Can you work these out from the model? Positions are in its coordinate system, mm. Coordinates: 2 decimals unless noted, no trailing zeros.
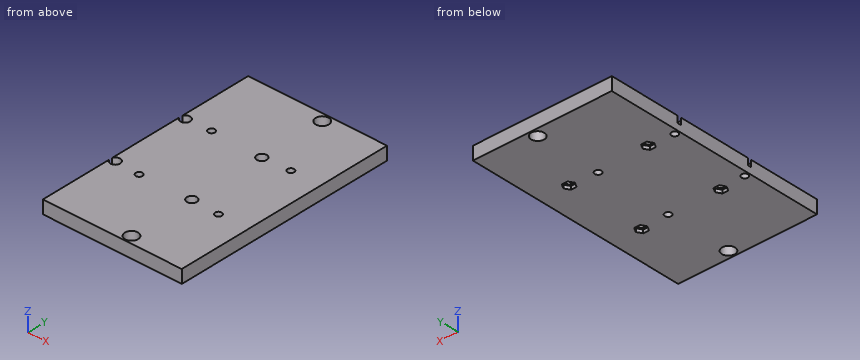
Autodesk Inventor part; units mm, degrees
ref_plane "YZ Plane" through (0, 0, 0) normal (1, 0, 0) x (0, 1, 0)
ref_plane "XZ Plane" through (0, 0, 0) normal (0, 1, 0) x (-1, 0, 0)
ref_plane "XY Plane" through (0, 0, 0) normal (0, 0, 1) x (1, 0, 0)
sketch "Sketch1" plane through (0, 0, 0) normal (0, 0, 1) x (1, 0, 0)
  line L0 (-33.3375, -53.975) -> (33.3375, -53.975)
  line L1 (33.3375, -53.975) -> (33.3375, 53.975)
  line L2 (33.3375, 53.975) -> (-33.3375, 53.975)
  line L3 (-33.3375, 53.975) -> (-33.3375, -53.975)
  line L4 (-33.3375, -53.975) -> (33.3375, 53.975) construction
  line L5 (33.3375, -53.975) -> (-33.3375, 53.975) construction
  point P0 (0, 0)
  dimension "d0" = 66.675
  dimension "d1" = 107.95
extrude "Extrusion1" add sketch "Sketch1" along normal blind 6.35
sketch "Sketch3" plane through (0, 0, 6.35) normal (0, 0, 1) x (1, 0, 0)
  line L0 (-19.05, -19.05) -> (19.05, -19.05)
  line L1 (19.05, -19.05) -> (19.05, 19.05)
  line L2 (19.05, 19.05) -> (-19.05, 19.05)
  line L3 (-19.05, 19.05) -> (-19.05, -19.05)
  line L4 (-19.05, -19.05) -> (19.05, 19.05) construction
  line L5 (19.05, -19.05) -> (-19.05, 19.05) construction
  line L6 (0, 0) -> (-12.7, 0)
  line L7 (-31.115, -18.415) -> (5.715, -18.415)
  line L8 (5.715, -18.415) -> (5.715, 18.415)
  line L9 (5.715, 18.415) -> (-31.115, 18.415)
  line L10 (-31.115, 18.415) -> (-31.115, -18.415)
  line L11 (-31.115, -18.415) -> (5.715, 18.415) construction
  line L12 (5.715, -18.415) -> (-31.115, 18.415) construction
  circle A0 centre (19.05, 19.05) radius 1.5875
  circle A1 centre (19.05, -19.05) radius 1.5875
  circle A2 centre (-19.05, 19.05) radius 1.5875
  circle A3 centre (-19.05, -19.05) radius 1.5875
  circle A4 centre (5.715, 18.415) radius 1.5875
  circle A5 centre (5.715, -18.415) radius 1.5875
  circle A6 centre (-31.115, 18.415) radius 1.5875
  circle A7 centre (-31.115, -18.415) radius 1.5875
  line L13 (5.715, 18.415) -> (5.715, 50.165)
  circle A8 centre (5.715, 50.165) radius 3.175
  line L14 (5.715, -18.415) -> (5.715, -50.165)
  circle A9 centre (5.715, -50.165) radius 3.175
  dimension "d11" = 38.1
  dimension "d12" = 38.1
  dimension "d13" = 12.7
  dimension "d14" = 36.83
  dimension "d15" = 36.83
  dimension "d16" = 3.175
  dimension "d17" = 3.175
  dimension "d18" = 3.175
  dimension "d19" = 3.175
  dimension "d20" = 3.175
  dimension "d21" = 3.175
  dimension "d22" = 3.175
  dimension "d23" = 3.175
  dimension "d24" = 31.75
  dimension "d25" = 6.35
  dimension "d26" = 31.75
  dimension "d27" = 6.35
extrude "Extrusion2" cut sketch "Sketch3" against normal blind 6.35 contours L3 L7 A3 L0 | L0 A3 L7 L3 | A8 | A9 | L7 A3 L3 | L3 A3 L7 | A5 L7 L14 L0 | L0 L14 A5 | L14 L8 A5 L0 | L0 A5 L14 | A5 L8 L7 | A7 L10 L7 | L7 L10 A7 | A2 L9 L3 | L3 L9 A2 | L9 A2 L2 L3 | L3 L2 A2 L9 | A1 L1 L0 | L0 L1 A1 | A4 L9 L8 | L8 L13 L2 A4 | A6 L9 L10 | L10 L9 A6 | A4 L2 L13 L9 | A4 L13 L2 | A0 L2 L1 | L1 L2 A0 | L13 A4 L2
sketch "Sketch4" plane through (0, 0, 6.35) normal (0, 0, 1) x (1, 0, 0)
  circle A0 centre (-31.115, 18.415) radius 1.5875
  circle A1 centre (-31.115, -18.415) radius 1.5875
  circle A2 centre (5.715, -18.415) radius 1.5875
  circle A3 centre (5.715, 18.415) radius 1.5875
  circle A4 centre (-31.115, 18.415) radius 2.3812
  circle A5 centre (-31.115, -18.415) radius 2.3813
  circle A6 centre (5.715, -18.415) radius 2.3812
  circle A7 centre (5.715, 18.415) radius 2.3813
  point P0 (0, 0)
  dimension "d30" = 4.7625
  dimension "d31" = 4.7625
  dimension "d32" = 4.7625
  dimension "d33" = 4.7625
extrude "Extrusion3" cut sketch "Sketch4" against normal blind 3.175
sketch "Sketch5" plane through (0, 0, 0) normal (0, 0, -1) x (-1, 0, 0)
  circle A0 centre (19.05, 19.05) radius 1.5875
  circle A1 centre (19.05, -19.05) radius 1.5875
  circle A2 centre (-19.05, -19.05) radius 1.5875
  circle A3 centre (-19.05, 19.05) radius 1.5875
  line L0 (-16.3004, 19.05) -> (-17.6752, 16.6687)
  line L1 (-17.6752, 16.6687) -> (-20.4248, 16.6687)
  line L2 (-20.4248, 16.6687) -> (-21.7996, 19.05)
  line L3 (-21.7996, 19.05) -> (-20.4248, 21.4312)
  line L4 (-20.4248, 21.4312) -> (-17.6752, 21.4313)
  line L5 (-17.6752, 21.4313) -> (-16.3004, 19.05)
  line L6 (-33.3375, 53.975) -> (33.3375, 53.975)
  line L7 (-33.3375, -53.975) -> (-33.3375, 53.975)
  line L8 (-16.3004, -19.05) -> (-17.6752, -21.4313)
  line L9 (-17.6752, -21.4313) -> (-20.4248, -21.4313)
  line L10 (-20.4248, -21.4313) -> (-21.7996, -19.05)
  line L11 (-21.7996, -19.05) -> (-20.4248, -16.6688)
  line L12 (-20.4248, -16.6688) -> (-17.6752, -16.6687)
  line L13 (-17.6752, -16.6687) -> (-16.3004, -19.05)
  line L14 (21.7996, 19.05) -> (20.4248, 16.6687)
  line L15 (20.4248, 16.6687) -> (17.6752, 16.6687)
  line L16 (17.6752, 16.6687) -> (16.3004, 19.05)
  line L17 (16.3004, 19.05) -> (17.6752, 21.4312)
  line L18 (17.6752, 21.4312) -> (20.4248, 21.4312)
  line L19 (20.4248, 21.4312) -> (21.7996, 19.05)
  line L20 (21.7996, -19.05) -> (20.4248, -21.4313)
  line L21 (20.4248, -21.4313) -> (17.6752, -21.4313)
  line L22 (17.6752, -21.4313) -> (16.3004, -19.05)
  line L23 (16.3004, -19.05) -> (17.6752, -16.6688)
  line L24 (17.6752, -16.6688) -> (20.4248, -16.6688)
  line L25 (20.4248, -16.6688) -> (21.7996, -19.05)
  point P0 (0, 0)
  point P1 (-19.05, -19.05)
  point P2 (19.05, 19.05)
  point P3 (19.05, -19.05)
  dimension "d36" = 4.7625
  dimension "d39" = 38.1
  dimension "d42" = 38.1
extrude "Extrusion4" cut sketch "Sketch5" against normal blind 1.5875
properties part number "lidarCamMountv2" material "ABS Plastic"
1. Imagine slicing it at A-A on z = 4.25. Give the number of separate pieces and of enclosed holes in the cut face, then the cut area to 3 significant figures.
Completed:
separate pieces: 1
enclosed holes: 8
area: 7,030 mm2
2. Please list where these lines run through material, in increasing order: probe 1 along Y at (x, z) = (-19.05, 4.25) (1 decimal); probe 2 along X at (y, z) = (-19.05, 5); probe 3 along X at (y, z) = (-21, 1).
Completed:
probe 1: y = -54 to -20.6, -17.5 to 17.5, 20.6 to 54
probe 2: x = -28.82 to -20.64, -17.46 to 3.42, 8.01 to 17.46, 20.64 to 33.34
probe 3: x = -33.34 to -20.67, -17.43 to 17.43, 20.67 to 33.34
3. I'm going to push flat-ended pins straight in: pin 1 (6 mm diameter, centred on x = -31.115, y = -18.415, fed in from -Z); pin 2 (1.4 mm diameter, centred on x = 19, y = 20, fed in from -Z). Where does each tip first touch, or does it pass through?
Completed:
pin 1: stops at z = 0
pin 2: stops at z = 1.59
